The model under review builds one solid part; all positions refer to its coordinate system, in mm. A direction names the side the tool comes from. Coordinates: 2 decimals unless noted, no trailing zeros. Write each loop counter-clockwise with the first axis right and the second up, starting at its lowest first coordinate (ties: lowest second). Pieces come first, ordered by that corner, then holes. Notation, with made-up numbers: (25.5, 64.5) - (80.5, 64.5) arc R24 cw to (80.5, 98.5) - close; hole circle Ø4 at (-17.75, -35.75). An arc over 180 degrees is marked (long way). Put each result on its own line as item: value.
from build123d import *

# Parameters (mm, degrees)
BOSS_EXTRUDE1_DEPTH         = 16
BOSS_EXTRUDE2_DEPTH         = 1.8
M4_TAPPED_HOLE1_AT_2_COUNT  = 2
M4_TAPPED_HOLE1_AT_2_PITCH  = 38.006280301
M5_TAPPED_HOLE1_D           = 4.2
M5_TAPPED_HOLE1_CSINK_D     = 5.05
M5_TAPPED_HOLE1_CSINK_ANGLE = 90
CUT_EXTRUDE1_REACH          = 45.032


with BuildPart() as part:
    # Sketch2 → Boss-Extrude1 (new body)
    with BuildSketch(Plane(origin=(0, 0, 0), x_dir=(1, 0, 0), z_dir=(0, 1, 0))):
        with BuildLine():
            Line((2.56174761, 3.509758774), (-4.43825239, 3.509758774))
            Line((-4.43825239, 3.509758774), (-6.046178238, 3.509758774))
            ThreePointArc((-6.046178238, 3.509758774), (-6.455374166, 2.715838994), (-6.818907741, 1.9))
            Line((-6.818907741, 1.9), (-6.818907741, 0.05))
            Line((-6.818907741, 0.05), (-5.306541861, 0.05))
            Line((-5.306541861, 0.05), (15.777709192, 0.05))
            Line((15.777709192, 0.05), (15.777709192, 0))
            Line((15.777709192, 0), (18.671266747, -2.599889358))
            Line((18.671266747, -2.599889358), (18.671266747, -5.599889358))
            Line((18.671266747, -5.599889358), (15.777709192, -8.199778717))
            Line((15.777709192, -8.199778717), (15.777709192, -8.25))
            Line((15.777709192, -8.25), (-5.306541861, -8.25))
            Line((-5.306541861, -8.25), (-6.818907741, -8.25))
            Line((-6.818907741, -8.25), (-6.818907741, -10.1))
            ThreePointArc((-6.818907741, -10.1), (-6.455374166, -10.915838994), (-6.046178238, -11.709758774))
            Line((-6.046178238, -11.709758774), (-4.43825239, -11.709758774))
            Line((-4.43825239, -11.709758774), (2.56174761, -11.709758774))
            Line((2.56174761, -11.709758774), (2.56174761, -17.495983577))
            Line((2.56174761, -17.495983577), (2.56174761, -18.97321001))
            ThreePointArc((2.56174761, -18.97321001), (13.37493466, -18.80880594), (21.533094515, -11.709758774))
            Line((21.533094515, -11.709758774), (21.533094515, 3.509758774))
            ThreePointArc((21.533094515, 3.509758774), (13.37493466, 10.60880594), (2.56174761, 10.77321001))
            Line((2.56174761, 10.77321001), (2.56174761, 9.295983577))
            Line((2.56174761, 9.295983577), (2.56174761, 3.509758774))
        make_face()
    extrude(amount=BOSS_EXTRUDE1_DEPTH)

    # Sketch4 → Boss-Extrude2 (add)
    with BuildSketch(Plane(origin=(0, 0, 0), x_dir=(1, 0, 0), z_dir=(0, 1, 0))):
        with BuildLine():
            Line((-1.167494267, 15.710466074), (20.167494267, 15.710466074))
            ThreePointArc((20.167494267, 15.710466074), (32, -4.1), (20.167494267, -23.910466074))
            Line((20.167494267, -23.910466074), (-1.167494267, -23.910466074))
            ThreePointArc((-1.167494267, -23.910466074), (-13, -4.1), (-1.167494267, 15.710466074))
        make_face()
    extrude(amount=BOSS_EXTRUDE2_DEPTH)

    # Sketch8 → M4 Tapped Hole1 (revolve, cut)
    with BuildSketch(Plane(origin=(28.620732779, 1.8, 4.51846258), x_dir=(0, 0, 1), z_dir=(1, 0, 0))):
        Polygon((0, 0), (0, 1.8), (1.65, 1.8), (1.65, 0.375), (2.025, 0), align=None)
    m4_tapped_hole1 = revolve(axis=Axis((28.620732779, 8.15, 4.51846258), (0, -1, 0)), mode=Mode.SUBTRACT)

    # M4 Tapped Hole1 at 2: M4 Tapped Hole1 ×2
    with Locations(*[Vector(-0.9999991610523592, 0, -0.001295335700845017) * (i * M4_TAPPED_HOLE1_AT_2_PITCH) for i in range(1, M4_TAPPED_HOLE1_AT_2_COUNT)]):
        add(m4_tapped_hole1, mode=Mode.SUBTRACT)

    # M5 Tapped Hole1 (through all)
    with Locations(Plane(origin=(0, 0, -10.05), x_dir=(1, 0, 0), z_dir=(0, 0, -1))):
        with Locations((-1.823787651, -11.616172117)):
            CounterSinkHole(M5_TAPPED_HOLE1_D / 2, M5_TAPPED_HOLE1_CSINK_D / 2, counter_sink_angle=M5_TAPPED_HOLE1_CSINK_ANGLE)

    # Sketch25 → Cut-Extrude1 (cut, up to next)
    with BuildSketch(Plane(origin=(0, 16, 0), x_dir=(1, 0, 0), z_dir=(0, 1, 0)), mode=Mode.PRIVATE) as cut_extrude1_sk1:
        Polygon((15.777709192, 0), (18.671266747, -2.599889358), (18.671266747, -5.599889358), (15.777709192, -8.199778717), (15.777709192, -8.25), (2.821266747, -8.25), (2.821266747, 0.05), (15.777709192, 0.05), align=None)
    cut_extrude1_tool1 = extrude(cut_extrude1_sk1.sketch, amount=-CUT_EXTRUDE1_REACH, mode=Mode.PRIVATE) & part.part
    add(cut_extrude1_tool1.solids().sort_by_distance((10.307921, 16, 4.099986))[0], mode=Mode.SUBTRACT)


solid = part.part
1. Consider section C-C on y = 11. State the section outline as (x, z) points, plus the area to 3 significant figures.
Determined:
outline: (-6.82, -1.9) arc R15.75 ccw to (-6.05, -3.51) - (-3.83, -3.51) - (-3.83, -0.05) - (-6.82, -0.05) - close; (-6.82, 8.25) - (-3.83, 8.25) - (-3.83, 11.71) - (-6.05, 11.71) arc R15.75 ccw to (-6.82, 10.1) - close; (0.18, -3.51) - (2.56, -3.51) - (2.56, -10.77) arc R15.75 ccw to (21.53, -3.51) - (21.53, 11.71) arc R15.75 ccw to (2.56, 18.97) - (2.56, 11.71) - (0.18, 11.71) - (0.18, 8.25) - (15.78, 8.25) - (15.78, 8.2) - (18.67, 5.6) - (18.67, 2.6) - (15.78, 0) - (15.78, -0.05) - (0.18, -0.05) - close
area: 440 mm^2
2. Consider section D-D on z = 7.5. State the section outline as (x, y) points.
Determined:
outline: (-12.74, 0) - (2.82, 0) - (2.82, 1.8) - (-12.74, 1.8) - close; (16.56, 0) - (31.74, 0) - (31.74, 1.8) - (21.53, 1.8) - (21.53, 16) - (16.56, 16) - close
3. Consider section A-A on y = 5.75. State the section outline as (x, z) points, plus the area to 3 significant figures.
Determined:
outline: (-6.82, -1.9) arc R15.75 ccw to (-6.05, -3.51) - (2.56, -3.51) - (2.56, -10.77) arc R15.75 ccw to (21.53, -3.51) - (21.53, 11.71) arc R15.75 ccw to (2.56, 18.97) - (2.56, 11.71) - (-6.05, 11.71) arc R15.75 ccw to (-6.82, 10.1) - (-6.82, 8.25) - (15.78, 8.25) - (15.78, 8.2) - (18.67, 5.6) - (18.67, 2.6) - (15.78, 0) - (15.78, -0.05) - (-6.82, -0.05) - close
area: 468 mm^2
4. Machinability: for faces 5 (the cylindrical face through (13.23, 8.801, 18.863)), 6 (the cylindrical face through (13.519, 8.801, -10.553)), 7 (the flat face through (-6.819, 9, -1)), 8 (the cylindrical face through (-6.45, 8.8, -2.73)), which of the approach directions +Z, -Z, +X, -X, +Y, -Y give a long, thin tool a straight path to every point of the face, cutting with its end or side? Answer none if there is none.
Determined:
face 5: +Z, +Y
face 6: -Z, +Y
face 7: +Z, -Z, -X, +Y
face 8: -Z, -X, +Y
5. For pin 1 Ø2.5 at (x, y) = (-3.5, 10) entering from -Z; pin 2 Ø5 at (y, z) = (4.5, -3.5) entering from +X; pin 3 Ø6 at (x, z) = (22, -8) entering from +Y; pin 4 Ø6 at (y, z) = (7.5, 15) entering from -X, all flat-tipped, find the tip position at first contact; note any pin that passes through.
Determined:
pin 1: stops at z = -3.51
pin 2: stops at x = 21.53
pin 3: stops at y = 16
pin 4: stops at x = 2.56
6. To check wall thickness, follow probe 1 along Z at (x, y) = (7.5, 11.25); probe 2 along X at (y, z) = (14.25, 5.5). State the ranges of each line that lie inside material, in increasing order.
Determined:
probe 1: z = -11.65 to -0.05, 8.25 to 19.85
probe 2: x = 18.67 to 21.53
7. Consider section B-B on x = 12.5. State the section outline as (y, z) points, plus the area to 3 significant figures.
Determined:
outline: (0, -15.71) - (1.8, -15.71) - (1.8, -10.91) - (16, -10.91) - (16, -0.05) - (0, -0.05) - close; (0, 8.25) - (16, 8.25) - (16, 19.11) - (1.8, 19.11) - (1.8, 23.91) - (0, 23.91) - close
area: 365 mm^2
8. The part is to be moulded in two halves that separate along Y. For faces 1 (the flat face through (10, 16, -3)), 2 (the flat face through (2.821, 1, 4)), 3 (the cylindrical face through (-1.369, 13.666, -1.756)), 4 (the flat face through (10, 0, -1)), say which applies: +Y half, -Y half, draft (parallel to the pull), parting line (faces both ways), or undercut.
Determined:
face 1: +Y half
face 2: draft
face 3: undercut
face 4: -Y half
